Autodesk Inventor part; units mm, degrees
ref_plane "YZ Plane" through (0, 0, 0) normal (1, 0, 0) x (0, 1, 0)
ref_plane "XZ Plane" through (0, 0, 0) normal (0, 1, 0) x (-1, 0, 0)
ref_plane "XY Plane" through (0, 0, 0) normal (0, 0, 1) x (1, 0, 0)
sketch "Sketch1" plane through (0, 0, 0) normal (0, 1, 0) x (-1, 0, 0)
  line L0 (6.21, 11.0673) -> (-74.79, 11.0673)
  line L1 (-74.79, 11.0673) -> (-74.79, -80.9327)
  line L2 (-74.79, -80.9327) -> (6.21, -80.9327)
  line L3 (6.21, -80.9327) -> (6.21, 11.0673)
  point P0 (0, 0)
  dimension "d0" = 81
  dimension "d1" = 92
extrude "Extrusion1" add sketch "Sketch1" along normal blind 4
sketch "Sketch2" plane through (0, 4, 0) normal (0, 1, 0) x (1, 0, 0)
  line L0 (-6.21, -11.0673) -> (74.79, -11.0673)
  line L1 (-3.1343, -11.0673) -> (0.8657, -11.0673) construction
  line L2 (-6.21, 80.9327) -> (-6.21, -11.0673)
  line L3 (-2.21, -7.0673) -> (70.79, -7.0673)
  line L4 (70.79, -7.0673) -> (70.79, 76.9327)
  line L5 (70.79, 76.9327) -> (-2.21, 76.9327)
  line L6 (-2.21, 76.9327) -> (-2.21, -7.0673)
  line L7 (74.79, -11.0673) -> (74.79, 80.9327)
  line L8 (-6.21, -11.0673) -> (74.79, -11.0673)
  line L9 (74.79, -11.0673) -> (74.79, 80.9327)
  line L10 (74.79, 80.9327) -> (-6.21, 80.9327)
  line L11 (-6.21, 80.9327) -> (-6.21, -11.0673)
  line L12 (-6.21, 80.9327) -> (-6.21, -11.0673)
  line L13 (2.4089, -7.0673) -> (4.4089, -7.0673) construction
  line L14 (-2.21, -5.0673) -> (-0.21, -5.0673) construction
  line L15 (-0.21, -5.0673) -> (68.79, -5.0673)
  line L16 (68.79, -5.0673) -> (68.79, 74.9327)
  line L17 (68.79, 74.9327) -> (-0.21, 74.9327)
  line L18 (-0.21, 74.9327) -> (-0.21, -5.0673)
  point P0 (0, 0)
  dimension "d8" = 73
  dimension "d9" = 84
  dimension "d14" = 69
  dimension "d15" = 80
extrude "Extrusion2" add sketch "Sketch2" along normal blind 4 contours L6 L5 L4 L3
sketch "Sketch3" plane through (0, 4, 0) normal (0, 1, 0) x (1, 0, 0)
  line L0 (-6.21, 80.9327) -> (-6.21, -11.0673)
  line L1 (-6.21, 78.6108) -> (34.29, 78.6108)
  line L2 (74.79, -11.0673) -> (74.79, 80.9327)
  line L3 (34.29, 78.6108) -> (34.29, 76.9327)
  line L4 (70.79, 76.9327) -> (-2.21, 76.9327)
  line L5 (34.29, 76.9327) -> (30.79, 76.9327)
  line L6 (30.79, 76.9327) -> (34.29, 76.9327)
  line L7 (34.29, 76.9327) -> (37.79, 76.9327)
  line L8 (37.79, 76.9327) -> (37.79, 73.9327)
  line L9 (37.79, 73.9327) -> (30.79, 73.9327)
  line L10 (30.79, 73.9327) -> (30.79, 76.9327)
  point P0 (0, 0)
  dimension "d18" = 40.5
  dimension "d19" = 3.5
  dimension "d20" = 3.5
  dimension "d21" = 3.5
  dimension "d22" = 3
  dimension "d23" = 7
extrude "Extrusion3" cut sketch "Sketch3" against normal blind 4
sketch "Sketch4" plane through (0, 4, 0) normal (0, -1, 0) x (1, 0, 0)
  line L0 (30.79, -76.9327) -> (37.79, -76.9327)
  line L1 (30.79, -73.9327) -> (30.79, -74.9327)
  line L2 (37.79, -76.9327) -> (30.79, -76.9327)
  line L3 (30.79, -76.9327) -> (30.79, -74.9327)
  line L4 (30.79, -74.9327) -> (37.79, -74.9327)
  line L5 (37.79, -74.9327) -> (37.79, -76.9327)
  point P0 (0, 0)
extrude "Extrusion4" cut sketch "Sketch4" against normal blind 10
sketch "Sketch5" plane through (30.79, 4, -76.9327) normal (0, 0, 1) x (1, 0, 0)
  line L0 (7, -4) -> (0, -4)
  line L1 (0, 0) -> (0, -4)
  line L2 (7, -4) -> (0, -4)
  line L3 (0, -4) -> (0, 0)
  line L4 (0, 0) -> (7, 0)
  line L5 (7, 0) -> (7, -4)
  point P0 (-30.79, -4)
extrude "Extrusion5" cut sketch "Sketch5" against normal blind 10
fillet "Fillet1" radius 2 9 edges at (74.79, 2, 11.0673) (74.79, 0, -34.9327) (34.29, 0, 11.0673) (-6.21, 2, 11.0673) (-6.21, 0, -34.9327) (-6.21, 2, -80.9327) (12.29, 0, -80.9327) (56.29, 0, -80.9327) (74.79, 2, -80.9327)
properties part number "Battery Box Lid_3DPrint"
Part model, mm, in its own coordinate system. A direction names the side the tool comes from. Give positions to 0.01 mm unless a question says otherwise; leave off trailing zeros. Order: outer loops, then holes, each group sorted by start corner. A loop starts at its lowest first (then second) coordinate and runs counter-clockwise, first axis right, second up. Notation, with made-up numbers: M 7.25,62 L 57.25,62 A20 cw 57.25,96 Z; hole C 62,-10.5 d3. An arc over 180 degrees is marked long. Use a Markdown table: item, result. Add a question column.
(1) Drop flat-ended pins along their axis: P1, Ø4.5, axis at x = 49.5, y = 6.5, coming from the -Z side; P2, Ø6, axis at x = 65, z = -34.5, coming from the +Y side; P3, Ø4.5, axis at x = 9, y = 5.5, coming from the -Z side; P4, Ø2, axis at x = 34, y = 1, coming from the -Z side. Give the stop position or say it passes through.
(2) Saw through at B-B, the plane x = 67. Give the cut face in (y, z), and give its area (3 significant figures).
(3) Saw through at C-C, the plane z = -18.5. Give the cut face in (x, y).
(4) Saw through at A-A, the plane y = 6. Give the cut face in (x, z), and give its area (3 significant figures).
(5) Probe line 1 along Z through (x, y) = (59.5, 7.5); line 2 along X through (y, z) = (7, -53); line 3 along X through (y, z) = (4.25, -75). List the from-to ranges inside material, lowest first. Write a range as [from, to].
(6) 3-axis set-ups, long thin cutter, end or side, ignore diameter. For faces 1 (the face through (16, 6, -74.933)), 2 (the face through (70.79, 6, -34)), 3 (the face through (30.79, 3, -77)), 4 (the face through (15, 6, -76.933)), 5 (the face through (-6.21, 3, -36)): which of +Z, -Z, +X, -X, +Y, -Y reach the whole face in a straight line?
(7) Mould opens along X. For faces 6 (the face through (-5.64, 3.014, 10.466)), 7 (the face through (-1, 8, -35)), 8 (the face through (34, 2, -73.933)), 9 (the face through (74.79, 3, -34)) say: +X half, -X half, draft (parallel to the pull), parting line (faces both ways), or undercut.
Answer key:
| question | item | result |
|---|---|---|
| 1 | P1 | z = -76.93 |
| 1 | P2 | y = 4 |
| 1 | P3 | z = -80.93 |
| 1 | P4 | z = -73.93 |
| 2 | outline | M 0,-78.93 A2 ccw 2,-80.93 L 4,-80.93 L 4,-76.93 L 8,-76.93 L 8,-74.93 L 4,-74.93 L 4,5.07 L 8,5.07 L 8,7.07 L 4,7.07 L 4,11.07 L 2,11.07 A2 ccw 0,9.07 Z |
| 2 | area | 382 mm^2 |
| 3 | outline | M -6.21,2 A2 ccw -4.21,0 L 72.79,0 A2 ccw 74.79,2 L 74.79,4 L 70.79,4 L 70.79,8 L 68.79,8 L 68.79,4 L -0.21,4 L -0.21,8 L -2.21,8 L -2.21,4 L -6.21,4 Z |
| 4 | outline | M -2.21,-76.93 L 30.79,-76.93 L 30.79,-74.93 L -0.21,-74.93 L -0.21,5.07 L 68.79,5.07 L 68.79,-74.93 L 37.79,-74.93 L 37.79,-76.93 L 70.79,-76.93 L 70.79,7.07 L -2.21,7.07 Z |
| 4 | area | 598 mm^2 |
| 5 | line 1 | [-76.93, -74.93], [5.07, 7.07] |
| 5 | line 2 | [-2.21, -0.21], [68.79, 70.79] |
| 5 | line 3 | [-2.21, 30.79], [37.79, 70.79] |
| 6 | face 1 | +Y |
| 6 | face 2 | +Z, -Z, +X, +Y |
| 6 | face 3 | -Z, +Y, -Y |
| 6 | face 4 | -Z, +X, -X, +Y |
| 6 | face 5 | +Z, -Z, -X, +Y, -Y |
| 7 | face 6 | -X half |
| 7 | face 7 | draft |
| 7 | face 8 | undercut |
| 7 | face 9 | +X half |
